Here's how the part is built. I have some questions about the finished solid (model axes, mm). Round coordinates to 2 decimals unless told otherwise and drop trailing zeros. Write each loop counter-clockwise with the first axis right and the second up, starting at its lowest first coordinate (ties: lowest second). Pieces come first, ordered by that corner, then holes. Notation, with made-up numbers: (-14, 70) -> (17, 70) arc R25 cw to (17, 93) -> close; hole circle Ø4 at (74, 13). An arc over 180 degrees is marked (long way). Answer as CSV lines item,"result".
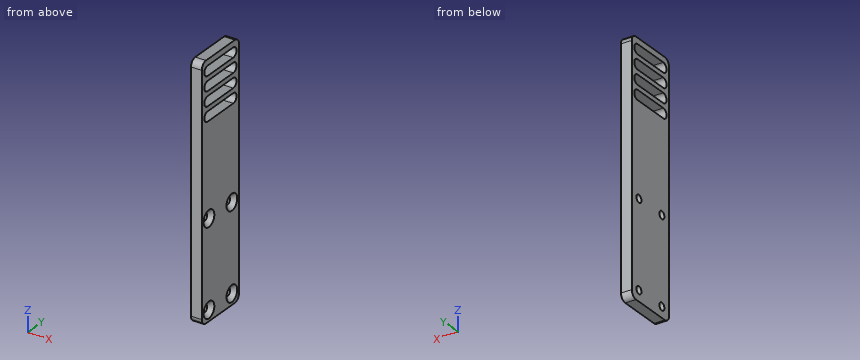
Autodesk Fusion 360 part; units mm, degrees
sketch "Sketch1" plane through (0, 0, 0) normal (1, 0, 0) x (0, 1, 0)
  line L0 (-13, 57.5) -> (13, 57.5)
  line L1 (13, 57.5) -> (13, -57.5)
  line L2 (13, -57.5) -> (-13, -57.5)
  line L3 (-13, -57.5) -> (-13, 57.5)
  line L4 (-13, 57.5) -> (13, -57.5) construction
  line L5 (13, 57.5) -> (-13, -57.5) construction
  circle A0 centre (-8, -12.5) radius 1.75
  circle A1 centre (8, -12.5) radius 1.75
  circle A2 centre (8, -52.5) radius 1.75
  circle A3 centre (-8, -52.5) radius 1.75
  line L6 (-9, 30.25) -> (9, 30.25)
  arc A4 (9, 30.25) -> (9, 34.75) centre (9, 32.5) ccw
  line L7 (9, 34.75) -> (-9, 34.75)
  arc A5 (-9, 34.75) -> (-9, 30.25) centre (-9, 32.5) ccw
  line L8 (-9, 32.5) -> (9, 32.5) construction
  line L9 (0, 0) -> (0, 10)
  arc A6 (-9, 41.4167) -> (-9, 36.9167) centre (-9, 39.1667) ccw
  line L10 (9, 41.4167) -> (-9, 41.4167)
  line L11 (-9, 39.1667) -> (9, 39.1667) construction
  line L12 (-9, 36.9167) -> (9, 36.9167)
  arc A7 (9, 36.9167) -> (9, 41.4167) centre (9, 39.1667) ccw
  arc A8 (-9, 48.0833) -> (-9, 43.5833) centre (-9, 45.8333) ccw
  line L13 (9, 48.0833) -> (-9, 48.0833)
  line L14 (-9, 45.8333) -> (9, 45.8333) construction
  line L15 (-9, 43.5833) -> (9, 43.5833)
  arc A9 (9, 43.5833) -> (9, 48.0833) centre (9, 45.8333) ccw
  arc A10 (-9, 54.75) -> (-9, 50.25) centre (-9, 52.5) ccw
  line L16 (9, 54.75) -> (-9, 54.75)
  line L17 (-9, 52.5) -> (9, 52.5) construction
  line L18 (-9, 50.25) -> (9, 50.25)
  arc A11 (9, 50.25) -> (9, 54.75) centre (9, 52.5) ccw
  dimension "d1" = 16
  dimension "d2" = 40
  dimension "d3" = 3.5
  dimension "d4" = 5
  dimension "d5" = 8
  dimension "d6" = 5
  dimension "d7" = 70
  dimension "d9" = 4.5
  dimension "d10" = 45
  dimension "d11" = 9
  dimension "d12" = 18
  dimension "d15" = 20
  dimension "d16" = 0
extrude "Extrude1" add sketch "Sketch1" along normal blind 5
fillet "Fillet1" radius 3 4 edges at (2.5, -13, 57.5) (2.5, 13, 57.5) (2.5, -13, -57.5) (2.5, 13, -57.5)
chamfer "Chamfer1" distance 2 angle 45 1 edges at (5, -9.6316, -11.8672)
chamfer "Chamfer1" distance 2 angle 45 3 edges at (5, 6.3684, -11.8672) (5, -9.6316, -51.8672) (5, 6.3684, -51.8672)
equation "d5 = ( 16 / 2 ) * 1 mm"
1. If I drill on line 1 (Z direction, x = 3.55, y = 4.75); line 2 (Z direction, x = 4.1, y = 11); line 3 (Y direction, x = 0.7, z = 39), over which ranges is the centre line in solid material (lowest first)?
Numbers:
line 1,"z = -57.5 to 30.25, 34.75 to 36.92, 41.42 to 43.58, 48.08 to 50.25, 54.75 to 57.5"
line 2,"z = -57.33 to 31.47, 33.53 to 38.14, 40.2 to 44.8, 46.86 to 51.47, 53.53 to 57.33"
line 3,"y = -13 to -11.24, 11.24 to 13"
2. Suppose I cut it at A-A on y = 8. Count the separate pieces of the cut face and the enclosed holes in it, and give its area (3 significant figures).
Numbers:
separate pieces,"7"
enclosed holes,"0"
area,"442 mm^2"
3. Suppose I cut it at B-B on z = 52.5. Please give me the cut outline in (x, y).
Numbers:
outline,"(0, -13) -> (5, -13) -> (5, -11.25) -> (0, -11.25) -> close; (0, 11.25) -> (5, 11.25) -> (5, 13) -> (0, 13) -> close"
4. Suppose I cut it at D-D on y = 2.5. Please give me the cut outline in (x, z), and give its area (3 significant figures).
Numbers:
outline,"(0, -57.5) -> (5, -57.5) -> (5, 30.25) -> (0, 30.25) -> close; (0, 34.75) -> (5, 34.75) -> (5, 36.92) -> (0, 36.92) -> close; (0, 41.42) -> (5, 41.42) -> (5, 43.58) -> (0, 43.58) -> close; (0, 48.08) -> (5, 48.08) -> (5, 50.25) -> (0, 50.25) -> close; (0, 54.75) -> (5, 54.75) -> (5, 57.5) -> (0, 57.5) -> close"
area,"485 mm^2"
